```python
from build123d import *


with BuildPart() as f1:
    # F0 (on Front) → F1 (revolve)
    with BuildSketch(Plane.XZ):
        with BuildLine():
            Line((0, 28), (0, 0))
            Line((0, 0), (5, 0))
            Line((5, 0), (5, 3.15))
            Line((5, 3.15), (12.2, 3.15))
            Line((12.2, 3.15), (12.2, 5.1))
            Line((12.2, 5.1), (15, 5.1))
            Line((15, 5.1), (15, 15))
            Line((15, 15), (13.762285, 22.019429))
            Line((13.762285, 22.019429), (9.732051, 29))
            ThreePointArc((9.732051, 29), (9, 29.732051), (8, 30))
            Line((8, 30), (7, 30))
            Line((7, 30), (5, 28))
            Line((5, 28), (3, 30))
            Line((3, 30), (2, 30))
            ThreePointArc((2, 30), (0.585786, 29.414214), (0, 28))
        make_face()
    revolve(axis=Axis((2.5, 0, 0), (-1, 0, 0)))


solid = f1.part
```
Here's how the part is built. I have some questions about the finished solid (model axes, mm). A direction names the side the tool comes from. Coordinates: 2 decimals unless noted, no trailing zeros. Write each loop counter-clockwise with the first axis right and the second up, starting at its lowest first coordinate (ties: lowest second). Pieces come first, ordered by that corner, then holes. Notation, with made-up numbers: M -27,-18 L 22,-18 A24 ccw 22,8 Z; hole C 67.25,18 d5. An arc over 180 degrees is marked long. Answer as CSV lines item,"result". Start each with the question number.
Q1. Suppose I cut it at A-A, the plane y = 0. List the corners of the cut face in (x, z) for me.
Q2. Will these pins go through, and if not, where does the flat tip stop? pin 1 Ø7 at (y, z) = (0, 0) entering from +X; pin 2 Ø2 at (x, z) = (8.5, 7) entering from +Y; pin 3 Ø1.9 at (y, z) = (-0.5, -0.5) entering from +X.
Q3. I need wall thicknesses on probe 1 along Y at (x, z) = (8, 0); probe 2 along Y at (x, z) = (6.75, 0); probe 3 along Z at (x, y) = (12.5, -4.5). Which ranges of each line are inside material? Lowest first, please. Write a range as [from, to].
Q4. If we mould it in two halves opening along Y, with no side actions, what happens to faces 4 (the flat face through (5, 0, 0)), 5 (the flat face through (15, -6, 0)), 6 (the conical face through (14.923, -15.072, -3.347))? For each: pulls with the +Y half, pulls with the -Y half, needs draft (parallel to the pull), parting line crosses it, or undercut.
Q5. For faces 1 (the conical face through (4.87, 8.45, 26.83)), 2 (the flat face through (12.2, 0.1, -3.3)), 3 (the cylindrical face through (7.49, 1.32, -29.97)), which set-ups out of +Z, -Z, +X, -X, +Y, -Y let a thin tool reach every point of the face, with its end or its side?
Entries:
1,outline,"M 0,-28 A2 ccw 2,-30 L 3,-30 L 5,-28 L 7,-30 L 8,-30 A2 ccw 9.73,-29 L 13.76,-22.02 L 15,-15 L 15,-5.1 L 12.2,-5.1 L 12.2,-3.15 L 5,-3.15 L 5,3.15 L 12.2,3.15 L 12.2,5.1 L 15,5.1 L 15,15 L 13.76,22.02 L 9.73,29 A2 ccw 8,30 L 7,30 L 5,28 L 3,30 L 2,30 A2 ccw 0,28 Z"
2,pin 1,"stops at x = 12.2"
2,pin 2,"stops at y = 29.38"
2,pin 3,"stops at x = 5"
3,probe 1,"y = [-30, -3.15], [3.15, 30]"
3,probe 2,"y = [-29.75, -3.15], [3.15, 29.75]"
3,probe 3,"z = [-23.78, -2.4], [2.4, 23.78]"
4,face 4,"undercut"
4,face 5,"needs draft"
4,face 6,"parting line crosses it"
5,face 1,"none"
5,face 2,"+X"
5,face 3,"+X, -X"
